from build123d import *

# Parameters (mm, degrees)
SKETCH1_W           = 55
SKETCH1_H           = 35
SKETCH1_R           = 1.75
BOSS_EXTRUDE1_DEPTH = 3
FILLET1_R           = 3
SKETCH2_W           = 49.2
SKETCH2_H           = 26
BOSS_EXTRUDE2_DEPTH = 21
FILLET2_R           = 13
BOSS_EXTRUDE3_DEPTH = 28.6
SKETCH4_R           = 3
CUT_EXTRUDE1_DEPTH  = 45.02888434
CUT_EXTRUDE2_DEPTH  = 16.05
SKETCH6_R           = 11.25
BOSS_EXTRUDE4_DEPTH = 8
SKETCH7_R           = 7.5
BOSS_EXTRUDE5_DEPTH = 8
FILLET3_R           = 1.5


with BuildPart() as part:
    # Sketch1 → Boss-Extrude1 (new body)
    with BuildSketch(Plane(origin=(0, 0, 0), x_dir=(1, 0, 0), z_dir=(0, 1, 0))):
        Rectangle(SKETCH1_W, SKETCH1_H)
        with Locations(Location((-23, 13, 0), (0, 0, 270))):
            Circle(SKETCH1_R, mode=Mode.SUBTRACT)
        with Locations(Location((-23, -13, 0), (0, 0, 270))):
            Circle(SKETCH1_R, mode=Mode.SUBTRACT)
        with Locations(Location((23, -13, 0), (0, 0, 270))):
            Circle(SKETCH1_R, mode=Mode.SUBTRACT)
        with Locations(Location((23, 13, 0), (0, 0, 270))):
            Circle(SKETCH1_R, mode=Mode.SUBTRACT)
    extrude(amount=BOSS_EXTRUDE1_DEPTH)

    # Fillet1
    fillet1_edges = [part.edges().sort_by_distance(p)[0] for p in [
        (27.5, 1.5, 17.5),
        (-27.5, 1.5, 17.5),
        (-27.5, 1.5, -17.5),
        (27.5, 1.5, -17.5),
    ]]
    fillet(fillet1_edges, radius=FILLET1_R)

    # Sketch2 → Boss-Extrude2 (add)
    with BuildSketch(Plane(origin=(0, 3, 0), x_dir=(1, 0, 0), z_dir=(0, 1, 0))):
        Rectangle(SKETCH2_W, SKETCH2_H)
    extrude(amount=BOSS_EXTRUDE2_DEPTH)

    # Fillet2
    # the kernel refuses this fillet: 13 mm, written as the material it takes off along each edge
    with BuildSketch(Plane(origin=(-24.6, 3, 13), x_dir=(1, 0, 0), z_dir=(0, 1, 0)), Plane(origin=(24.6, 3, -13), x_dir=(-1, 0, 0), z_dir=(0, 1, 0)), Plane(origin=(24.6, 3, 13), x_dir=(0, 0, -1), z_dir=(0, 1, 0))) as fillet2_piece_1:
        with BuildLine():
            CenterArc((FILLET2_R, FILLET2_R), FILLET2_R, 180, 90)
            Line((0, FILLET2_R), (0, 0))
            Line((0, 0), (FILLET2_R, 0))
        make_face()
    extrude(amount=53.5, mode=Mode.SUBTRACT)
    with BuildSketch(Plane(origin=(-24.6, 3, -13), x_dir=(1, 0, 0), z_dir=(0, 1, 0))) as fillet2_piece_2:
        with BuildLine():
            CenterArc((FILLET2_R, -FILLET2_R), FILLET2_R, 90, 90)
            Line((0, -FILLET2_R), (0, 0))
            Line((0, 0), (FILLET2_R, 0))
        make_face()
    extrude(amount=53.5, mode=Mode.SUBTRACT)

    # Sketch3 → Boss-Extrude3 (add)
    with BuildSketch(Plane.XZ):
        Polygon((-11, 0), (-17, 0), (-17, -1.5875), (-5, -1.5875), (-5, 0), align=None)
        Polygon((-17, 1.5875), (-17, 0), (-11, 0), (-5, 0), (-5, 1.5875), align=None)
        Polygon((5, 1.5875), (5, 0), (11, 0), (17, 0), (17, 1.5875), align=None)
        Polygon((11, 0), (5, 0), (5, -1.5875), (17, -1.5875), (17, 0), align=None)
    extrude(amount=BOSS_EXTRUDE3_DEPTH)

    # Sketch4 → Cut-Extrude1 (cut, through all)
    with BuildSketch(Plane.XY.offset(1.5875)):
        with Locations((-11, -22.1)):
            Circle(SKETCH4_R)
    cut_extrude1 = extrude(amount=-CUT_EXTRUDE1_DEPTH, mode=Mode.SUBTRACT)

    # Mirror1: Cut-Extrude1 across plane
    add(cut_extrude1.mirror(Plane(origin=(0, 0, 0), x_dir=(0, 0, 1), z_dir=(1, 0, 0))), mode=Mode.SUBTRACT)

    # Sketch5 → Cut-Extrude2 (cut)
    with BuildSketch(Plane(origin=(0, 24, 0), x_dir=(1, 0, 0), z_dir=(0, 1, 0))):
        with BuildLine():
            Line((-11.6, -10), (11.6, -10))
            ThreePointArc((11.6, -10), (18.671067812, -7.071067812), (21.6, 0))
            ThreePointArc((21.6, 0), (18.671067812, 7.071067812), (11.6, 10))
            Line((11.6, 10), (-11.6, 10))
            ThreePointArc((-11.6, 10), (-18.671067812, 7.071067812), (-21.6, 0))
            ThreePointArc((-21.6, 0), (-18.671067812, -7.071067812), (-11.6, -10))
        make_face()
    extrude(amount=-CUT_EXTRUDE2_DEPTH, mode=Mode.SUBTRACT)

    # Sketch6 → Boss-Extrude4 (add)
    with BuildSketch(Plane.XZ):
        with BuildLine():
            Line((-11, 1.5875), (-11, 11.25))
            ThreePointArc((-11, 11.25), (-22.25, 0), (-11, -11.25))
            Line((-11, -11.25), (-11, -1.5875))
            Line((-11, -1.5875), (-17, -1.5875))
            Line((-17, -1.5875), (-17, 1.5875))
            Line((-17, 1.5875), (-11, 1.5875))
        make_face()
        with BuildLine():
            ThreePointArc((0, 2.358495283), (-3.927891825, 8.749159158), (-11, 11.25))
            Line((-11, 11.25), (-11, 1.5875))
            Line((-11, 1.5875), (-5, 1.5875))
            Line((-5, 1.5875), (-5, -1.5875))
            Line((-5, -1.5875), (-11, -1.5875))
            Line((-11, -1.5875), (-11, -11.25))
            ThreePointArc((-11, -11.25), (-3.927891825, -8.749159158), (0, -2.358495283))
            ThreePointArc((0, -2.358495283), (-0.25, 0), (0, 2.358495283))
        make_face()
        with BuildLine():
            Line((11, 1.5875), (11, 11.25))
            ThreePointArc((11, 11.25), (3.927891825, 8.749159158), (0, 2.358495283))
            ThreePointArc((0, 2.358495283), (0.187325418, 1.185854123), (0.25, 0))
            ThreePointArc((0.25, 0), (0.187325418, -1.185854123), (0, -2.358495283))
            ThreePointArc((0, -2.358495283), (3.927891825, -8.749159158), (11, -11.25))
            Line((11, -11.25), (11, -1.5875))
            Line((11, -1.5875), (5, -1.5875))
            Line((5, -1.5875), (5, 1.5875))
            Line((5, 1.5875), (11, 1.5875))
        make_face()
        with BuildLine():
            ThreePointArc((22.25, 0), (18.954951288, 7.954951288), (11, 11.25))
            Line((11, 11.25), (11, 1.5875))
            Line((11, 1.5875), (17, 1.5875))
            Line((17, 1.5875), (17, -1.5875))
            Line((17, -1.5875), (11, -1.5875))
            Line((11, -1.5875), (11, -11.25))
            ThreePointArc((11, -11.25), (18.954951288, -7.954951288), (22.25, 0))
        make_face()
        with BuildLine():
            ThreePointArc((0, 2.358495283), (3.927891825, 8.749159158), (11, 11.25))
            Line((11, 11.25), (-11, 11.25))
            ThreePointArc((-11, 11.25), (-3.927891825, 8.749159158), (0, 2.358495283))
        make_face()
        with BuildLine():
            ThreePointArc((0, -2.358495283), (-3.927891825, -8.749159158), (-11, -11.25))
            Line((-11, -11.25), (11, -11.25))
            ThreePointArc((11, -11.25), (3.927891825, -8.749159158), (0, -2.358495283))
        make_face()
        with Locations((11, 0)):
            Circle(SKETCH6_R)
        with Locations((-11, 0)):
            Circle(SKETCH6_R)
    extrude(amount=BOSS_EXTRUDE4_DEPTH)

    # Sketch7 → Boss-Extrude5 (add)
    with BuildSketch(Plane(origin=(0, 7.95, 0), x_dir=(1, 0, 0), z_dir=(0, 1, 0))):
        with Locations(Location((-11, 0, 0), (0, 0, 270))):
            Circle(SKETCH7_R)
        with Locations(Location((11, 0, 0), (0, 0, 270))):
            Circle(SKETCH7_R)
    extrude(amount=BOSS_EXTRUDE5_DEPTH)

    # Fillet3
    fillet3_edges = [part.edges().sort_by_distance(p)[0] for p in [
        (-5, -28.6, 0),
        (-17, -28.6, 0),
        (17, -28.6, 0),
        (5, -28.6, 0),
    ]]
    fillet(fillet3_edges, radius=FILLET3_R)


solid = part.part
Source: CAD feature listing. Evaluate the final solid. Frame: model axes, mm. A direction names the side the tool comes from. Round coordinates to 2 decimals unless told otherwise and drop trailing zeros. Loops run counter-clockwise (first coordinate to the right, second up) from the corner with the lowest first, then second, coordinate; pieces in that order, holes last. Notation, with made-up numbers: (-20, 39.25) - (30, 39.25) arc R10 cw to (30, 46.25) - close; hole circle Ø9 at (11, -25.5). An arc over 180 degrees is marked (long way). Write item = value, one per line. Start each with the question number.
(1) Set-up query: faces 4 (the face through (0, 16, 10)), 5 (the face through (24.597, 13.353, 0.286)), 6 (the face through (-22.247, -3.944, 0.247)), 7 (the face through (5, -17, 0)). Return all of +Z, -Z, +X, -X, +Y, -Y with unobstructed straight access to the full face (end or side cutting, diameter ignored); none if empty.
(2) Section query A-A, the plane y = 12. Output: boundary loops of the cut face in (x, z), plus the area to 3 significant figures.
(3) Section query C-C, the plane x = 23. Output: boundary loops of the cut face in (y, z).
(4) Ray query, line 1 along Z through (x, y) = (23, 1); line 2 along X through (y, z) = (1.85, -13); line 3 along Y through (x, z) = (-17.5, -12). Return the intervals inside material, ascending. Write a range as from..to.
(5) Section query B-B, the plane y = 2. Output: boundary loops of the cut face in (x, z), plus the area to 3 significant figures.
(6) Pin query (flat end, axial travel): pin 1 (1.5 mm diameter, centred on x = 9, y = -5.5, fed in from +Z); pin 2 (17 mm diameter, centred on x = 3, y = 16.5, fed in from +Z); pin 3 (3.5 mm diameter, centred on y = -19, z = 1, fed in from -X); pin 4 (16.5 mm diameter, centred on x = -12, z = -3, fed in from +Y). Return the tip coordinate at first contact, or that it passes through.
(7) Pull-direction query (X, two-part tool) for faces 1 (the face through (-11, -18, 1.588)), 2 (the face through (-26.64, 1.52, -16.6)), 3 (the face through (11.65, -25.03, 0.02)); classes: +X half, -X half, draft (parallel to the pull), parting line (faces both ways), or undercut.
(8) Section query D-D, the plane y = -24. Output: boundary loops of the cut face in (x, z), plus the area to 3 significant figures.
Conclusion:
q1.face_4 = +Y
q1.face_5 = +X, +Y
q1.face_6 = -X, -Y
q1.face_7 = +Z, -Z, -Y
q2.outline = circle Ø15 at (-11, 0); (-11.6, -13) - (11.6, -13) arc R13 ccw to (11.6, 13) - (-11.6, 13) arc R13 ccw to start; circle Ø15 at (11, 0); hole (-11.6, -10) - (11.6, -10) arc R10 ccw to (11.6, 10) - (-11.6, 10) arc R10 ccw to start
q2.area = 709 mm2
q3.outline = (0, -17.5) - (3, -17.5) - (3, -14.75) - (0, -14.75) - close; (0, -11.25) - (3, -11.25) - (3, -6.25) - (24, -6.25) - (24, 6.25) - (3, 6.25) - (3, 11.25) - (0, 11.25) - close; (0, 14.75) - (3, 14.75) - (3, 17.5) - (0, 17.5) - close
q4.line_1 = -17.5..-14.75, -11.25..11.25, 14.75..17.5
q4.line_2 = -27.5..-24.75, -21.25..21.25, 24.75..27.5
q4.line_3 = 0..3
q5.outline = (-27.5, -14.5) arc R3 ccw to (-24.5, -17.5) - (24.5, -17.5) arc R3 ccw to (27.5, -14.5) - (27.5, 14.5) arc R3 ccw to (24.5, 17.5) - (-24.5, 17.5) arc R3 ccw to (-27.5, 14.5) - close; hole circle Ø3.5 at (-23, -13); hole circle Ø3.5 at (-23, 13); hole circle Ø3.5 at (23, -13); hole circle Ø3.5 at (23, 13)
q5.area = 1,880 mm2
q6.pin_1 = 11.25
q6.pin_2 = 13
q6.pin_3 = -17
q6.pin_4 = 24
q7.face_1 = draft
q7.face_2 = -X half
q7.face_3 = undercut
q8.outline = (-17, -1.59) - (-13.32, -1.59) - (-13.32, 1.59) - (-17, 1.59) - close; (-8.68, -1.59) - (-5, -1.59) - (-5, 1.59) - (-8.68, 1.59) - close; (5, -1.59) - (8.68, -1.59) - (8.68, 1.59) - (5, 1.59) - close; (13.32, -1.59) - (17, -1.59) - (17, 1.59) - (13.32, 1.59) - close
q8.area = 46.7 mm2
